Autodesk Inventor part; units mm, degrees
ref_plane "YZ Plane" through (0, 0, 0) normal (1, 0, 0) x (0, 1, 0)
ref_plane "XZ Plane" through (0, 0, 0) normal (0, 1, 0) x (-1, 0, 0)
ref_plane "XY Plane" through (0, 0, 0) normal (0, 0, 1) x (1, 0, 0)
ref_plane "Work Plane1" through (0, 0, 0) normal (0, 0, 1) x (1, 0, 0)
sketch "Sketch1" plane through (0, 0, 0) normal (0, 0, 1) x (1, 0, 0)
  line L0 (30.375, 39.1) -> (-30.4, 39.1)
  arc A0 (34.375, 35.1014) -> (30.375, 39.1) centre (30.375, 35.1) ccw
  line L1 (34.4, -35.0986) -> (34.375, 35.1014)
  arc A1 (30.4, -39.1) -> (34.4, -35.0986) centre (30.4, -35.1) ccw
  line L2 (-30.375, -39.1) -> (30.4, -39.1)
  arc A2 (-34.375, -35.1014) -> (-30.375, -39.1) centre (-30.375, -35.1) ccw
  line L3 (-34.4, 35.0986) -> (-34.375, -35.1014)
  arc A3 (-30.4, 39.1) -> (-34.4, 35.0986) centre (-30.4, 35.1) ccw
  arc A4 (-35.875, -35.102) -> (-30.375, -40.6) centre (-30.375, -35.1) ccw
  line L4 (30.4, -40.6) -> (-30.375, -40.6)
  arc A5 (30.4, -40.6) -> (35.9, -35.098) centre (30.4, -35.1) ccw
  line L5 (35.875, 35.102) -> (35.9, -35.098)
  arc A6 (35.875, 35.102) -> (30.375, 40.6) centre (30.375, 35.1) ccw
  line L6 (-30.4, 40.6) -> (30.375, 40.6)
  arc A7 (-30.4, 40.6) -> (-35.9, 35.098) centre (-30.4, 35.1) ccw
  line L7 (-35.875, -35.102) -> (-35.9, 35.098)
  point P0 (0, 0)
extrude "Extrusion1" add sketch "Sketch1" along normal blind 27.93
sketch "Sketch2" plane through (0, 0, 27.93) normal (0, 0, 1) x (1, 0, 0)
  line L0 (-35.9, 35.098) -> (-35.875, -35.102)
  arc A0 (-35.875, -35.102) -> (-30.375, -40.6) centre (-30.375, -35.1) ccw
  line L1 (-30.375, -40.6) -> (30.4, -40.6)
  arc A1 (30.4, -40.6) -> (35.9, -35.098) centre (30.4, -35.1) ccw
  line L2 (35.9, -35.098) -> (35.875, 35.102)
  arc A2 (35.875, 35.102) -> (30.375, 40.6) centre (30.375, 35.1) ccw
  line L3 (30.375, 40.6) -> (-30.4, 40.6)
  arc A3 (-30.4, 40.6) -> (-35.9, 35.098) centre (-30.4, 35.1) ccw
  point P0 (0, 0)
extrude "Extrusion2" add sketch "Sketch2" along normal blind 2
sketch "Sketch3" plane through (-30.4, 40.6, 0) normal (0, 1, 0) x (1, 0, 0)
  line L0 (48.3031, -6.91) -> (17.8231, -6.91)
  line L1 (48.3031, -6.91) -> (48.3031, -18.01)
  line L2 (17.8231, -6.91) -> (17.8231, -18.01)
  line L3 (48.3031, -18.01) -> (17.8231, -18.01)
  line L4 (48.3031, -18.01) -> (32.3031, -18.01)
  line L5 (32.3031, -18.01) -> (32.3031, -6.91)
  point P0 (30.4, 0)
  dimension "d9" = 16
extrude "Extrusion3" cut sketch "Sketch3" against normal blind 7.45 contours L1 L3 L5 L0
sketch "Sketch4" plane through (-30.375, -40.6, 0) normal (0, -1, 0) x (1, 0, 0)
  line L0 (17.0619, 6.91) -> (17.0619, 18.01)
  line L1 (32.3019, 6.91) -> (17.0619, 6.91)
  line L2 (49.2019, 6.91) -> (33.9619, 6.91)
  line L3 (49.2019, 6.91) -> (49.2019, 18.01)
  line L4 (17.0619, 18.01) -> (49.2019, 18.01)
  line L5 (32.3019, 6.91) -> (33.9619, 6.91)
  line L6 (-0.025, 0) -> (60.75, 0)
  line L7 (49.4019, 18.21) -> (49.4019, 6.71)
  line L8 (49.4019, 6.71) -> (33.9619, 6.71)
  line L9 (33.9619, 6.71) -> (32.3019, 6.71)
  line L10 (32.3019, 6.71) -> (16.8619, 6.71)
  line L11 (16.8619, 6.71) -> (16.8619, 18.21)
  line L12 (16.8619, 18.21) -> (49.4019, 18.21)
  point P0 (30.375, 0)
  dimension "d6" = 0.2
extrude "Extrusion4" cut sketch "Sketch4" against normal blind 7.45 contours L0 L4 L3 L2 L5 L1 | L7 L8 L9 L10 L11 L12
The listing builds one solid part. Answer for the finished solid, in the listing's coordinates (mm). A direction names the side the tool comes from. Give positions to 0.01 mm unless a question says otherwise; leave off trailing zeros. Write each loop counter-clockwise with the first axis right and the second up, starting at its lowest first coordinate (ties: lowest second). Pieces come first, ordered by that corner, then holes.
1) Find the intervals of material crossed by L1, parallel to X at y = -6, z = 4.5; L2, parallel to Y at x = 10.5, z = 19; L3, parallel to Z at x = -12.5, y = 18, in increasing order.
2) Section C-C (x = 1) is taken. Write down the section's boundary in (y, z), and give its area (3 significant figures).
3) Section A-A (z = 16) is taken. Write down the section's boundary in (x, y) (3 decimals).
4) A tool of negligible diameter and unlimited length cuts with its end or side. For faces 4 (the face through (34.22, 39.03, 14.76)), 5 (the face through (-33.17, -37.96, 13.77)), from which of +Z, -Z, +X, -X, +Y, -Y can it reach the whole face along a straight path? Write none if from no direction.
5) For a pull along Y with two mould halves and no side action, classify faces 1 (the face through (0, 40.6, 15)), 2 (the face through (-33.26, 37.897, 13.769)), 3 (the face through (0, -40.6, 21)) as pulls with the +Y half, pulls with the -Y half, needs draft (parallel to the pull), parting line crosses it, or undercut.
6) Section D-D (z = 25.5) is taken. Write down the section's boundary in (x, y) (3 decimals), and give its area (3 significant figures).
7) Given P1, Ø10, axis at y = 5.5, z = 26.5, coming from the -X side; P2, Ø4, axis at y = -4, z = 25.5, coming from the +X side; P3, Ø1.2, axis at y = 39.5, z = 10.5, coming from the +X side; P4, Ø4, axis at x = 5, z = 13, coming from the +Y side, each flat-ended and moving along its own axis, determine where each tip first touches the part or whether it passes through.
8) Section B-B (x = 9) is taken. Write down the section's boundary in (y, z), and give its area (3 significant figures).
Response:
1. L1: x = -35.89 to -34.39, 34.39 to 35.89
1. L2: y = -40.6 to -39.1, 39.1 to 40.6
1. L3: z = 27.93 to 29.93
2. outline: (-40.6, 0) - (-39.1, 0) - (-39.1, 6.71) - (-40.6, 6.71) - close; (-40.6, 18.21) - (-39.1, 18.21) - (-39.1, 27.93) - (39.1, 27.93) - (39.1, 0) - (40.6, 0) - (40.6, 29.93) - (-40.6, 29.93) - close
2. area: 229 mm2
3. outline: (-35.9, 35.098) - (-35.875, -35.102) arc R5.5 ccw to (-30.375, -40.6) - (-13.513, -40.6) - (-13.513, -39.1) - (-30.375, -39.1) arc R4 cw to (-34.375, -35.101) - (-34.4, 35.099) arc R4 cw to (-30.4, 39.1) - (1.903, 39.1) - (1.903, 40.6) - (-30.4, 40.6) arc R5.5 ccw to start; (17.903, 39.1) - (30.375, 39.1) arc R4 cw to (34.375, 35.101) - (34.4, -35.099) arc R4 cw to (30.4, -39.1) - (19.027, -39.1) - (19.027, -40.6) - (30.4, -40.6) arc R5.5 ccw to (35.9, -35.098) - (35.875, 35.102) arc R5.5 ccw to (30.375, 40.6) - (17.903, 40.6) - close
4. face 4: +Z, -Z, +X, +Y
4. face 5: -Z
5. face 1: pulls with the +Y half
5. face 2: undercut
5. face 3: pulls with the -Y half
6. outline: (-35.9, 35.098) - (-35.875, -35.102) arc R5.5 ccw to (-30.375, -40.6) - (30.4, -40.6) arc R5.5 ccw to (35.9, -35.098) - (35.875, 35.102) arc R5.5 ccw to (30.375, 40.6) - (-30.4, 40.6) arc R5.5 ccw to start; hole (-34.4, 35.099) - (-34.375, -35.101) arc R4 ccw to (-30.375, -39.1) - (30.4, -39.1) arc R4 ccw to (34.4, -35.099) - (34.375, 35.101) arc R4 ccw to (30.375, 39.1) - (-30.4, 39.1) arc R4 ccw to start
6. area: 438 mm2
7. P1: stops at x = -35.89
7. P2: stops at x = 35.89
7. P3: stops at x = 34.35
7. P4: passes through
8. outline: (-40.6, 0) - (-39.1, 0) - (-39.1, 6.71) - (-40.6, 6.71) - close; (-40.6, 18.21) - (-39.1, 18.21) - (-39.1, 27.93) - (39.1, 27.93) - (39.1, 18.01) - (40.6, 18.01) - (40.6, 29.93) - (-40.6, 29.93) - close; (39.1, 0) - (40.6, 0) - (40.6, 6.91) - (39.1, 6.91) - close
8. area: 212 mm2
